Source: CAD feature listing. Evaluate the final solid. Frame: model axes, mm. A direction names the side the tool comes from. Round coordinates to 2 decimals unless told otherwise and drop trailing zeros. Loops run counter-clockwise (first coordinate to the right, second up) from the corner with the lowest first, then second, coordinate; pieces in that order, holes last. Notation, with made-up numbers: M 8,-6.5 L 48,-6.5 A23 cw 48,13.5 Z; hole C -10,62.25 d8. An arc over 180 degrees is marked long. Write each question's results on one line, items separated by ' | '. Start each with the question number.
1. Contact query for flat-ended pins moving along their axis: pin 1 Ø20 at (x, z) = (-3, 4) entering from +Y; pin 2 Ø17.5 at (x, z) = (-15, 15) entering from -Y; pin 3 Ø10 at (y, z) = (-3, 30.5) entering from +X; pin 4 Ø1 at (y, z) = (1, 3.5) entering from -X. Output: stop coordinate, or through.
2. Section A-A on z = 30. Output: boundary loops of the cut face in (x, y).
3. Draft query along Y for faces 5 (the flat face through (0, -9.4, 0)), 6 (the flat face through (-11, 5, 61)), 7 (the cylindrical face through (-1.472, -8.137, 4.674)), 8 (the flat face through (-11, -5, 61)). Return one class per face: released by +Y, released by -Y, zero draft, split by the parting line, or undercut.
4. Section B-B on x = -7. Output: boundary loops of the cut face in (y, z).
5. Set-up query: faces 1 (the flat face through (-2.92, 0.13, 17)), 2 (the flat face through (-8.988, 0.071, 13.305)), 3 (the flat face through (1, 0, 70)), 4 (the cylindrical face through (1.472, 7.763, 4.674)). Return all of +Z, -Z, +X, -X, +Y, -Y with unobstructed straight access to the full face (end or side cutting, diameter ignored); none if empty.
6. Ray query, line 1 (Y direction, x = -5.5, z = 16); line 2 (Y direction, x = -20, z = 50); line 3 (X direction, y = -6.6, z = 30). Return the intervals inside material, ascending.
7. Section C-C on z = 0. Output: boundary loops of the cut face in (x, y), and give its area (3 significant figures).
from build123d import *
from build123d.topology import SkipClean

# Parameters (mm, degrees)
EXTRUDE_1_DEPTH          = 6.8
SKETCH_2_R               = 10
EXTRUDE_1_2_DEPTH        = 14
EXTRUDE_START            = -9
EXTRUDE_2_DEPTH          = 18
CUT_EXTRUDE_1_DEPTH      = 5.1
SKETCH_5_R               = 4.9
EXTRUDE_3_DEPTH          = 15
SKETCH_6_R               = 5.15
CUT_EXTRUDE_5_DEPTH      = 20
CUT_EXTRUDE_8_DEPTH      = 5
CUT_EXTRUDE_8_DEPTH_BACK = 5
CUT_EXTRUDE_8_START      = -9
SKETCH_9_R               = 5.15
CUT_EXTRUDE_9_DEPTH      = 5
SKETCH_11_R              = 0.75
CUT_EXTRUDE_10_DEPTH     = 2
CUT_EXTRUDE_11_DEPTH     = 2
CUT_EXTRUDE_12_DEPTH     = 2
SKETCH_7_W               = 20.220207393
SKETCH_7_H               = 10
CUT_EXTRUDE_14_DEPTH     = 14
CHAMFER_C0_3_SIZE        = 0.3
SKETCH_19_R              = 4.9
EXTRUDE_9_8_2_2_DEPTH    = 2.2
CHAMFER_C0_3_2_SIZE      = 0.3


# Read off the part's stored shape, not the designer's step: the extrude step
with BuildPart() as part:
    # Sketch 1 → Extrude 1 (new, symmetric)
    with BuildSketch(Plane(origin=(0, 0, 0), x_dir=(1, 0, 0), z_dir=(0, 1, 0))):
        Polygon((-5.82435206, 3.882901374), (-27, -27.880570536), (-27, -58.585636208), (0.909866919, -78.68074039), (9.090133081, -67.31925961), (-13, -51.414363792), (-13, -32.119429464), (5.82435206, -3.882901374), align=None)
    extrude(amount=EXTRUDE_1_DEPTH, both=True)

    # Sketch 2 → Extrude 1 2 (add)
    with BuildSketch(Plane(origin=(0, 6.8, 0), x_dir=(1, 0, 0), z_dir=(0, 1, 0))):
        with Locations(Location((0, 0, 0), (0, 0, 270))):
            Circle(SKETCH_2_R)
        with Locations(Location((-20, -30, 0), (0, 0, 270))):
            Circle(SKETCH_2_R)
    extrude(amount=-EXTRUDE_1_2_DEPTH)

    # Extrude 2 outline → Extrude 2 (add)
    with SkipClean():  # the faces are left unmerged after this step: merging them gives an invalid solid
        with BuildSketch(Plane(origin=(0, 0, 0), x_dir=(1, 0, 0), z_dir=(0, 1, 0)).offset(EXTRUDE_START)):
            with BuildLine():
                Line((-14.730348136, -9.47609274), (-21.86300031, -20.175071))
                ThreePointArc((-21.86300031, -20.175071), (-29.570920265, -27.102158513), (-27, -37.141428429))
                Line((-27, -37.141428429), (-27, -58.585636208))
                Line((-27, -58.585636208), (0.909866919, -78.68074039))
                Line((0.909866919, -78.68074039), (9.090133081, -67.31925961))
                Line((9.090133081, -67.31925961), (-13, -51.414363792))
                Line((-13, -51.414363792), (-13, -37.141428429))
                ThreePointArc((-13, -37.141428429), (-10.429079735, -32.897841487), (-10.214296189, -27.940873748))
                Line((-10.214296189, -27.940873748), (-3.081644015, -17.241895487))
                Line((-3.081644015, -17.241895487), (-14.730348136, -9.47609274))
            make_face()
        extrude(amount=EXTRUDE_2_DEPTH)
    add(part.part.scale(1), mode=Mode.REPLACE)  # the faces are merged on a copy

    # Sketch 4 → Cut-Extrude 1 (cut, symmetric)
    with BuildSketch(Plane(origin=(0, 0, 0), x_dir=(1, 0, 0), z_dir=(0, 1, 0))):
        with BuildLine():
            Line((-13, -37.141428429), (-13, -43.141428429))
            Line((-13, -43.141428429), (-27, -43.141428429))
            Line((-27, -43.141428429), (-27, -37.141428429))
            ThreePointArc((-27, -37.141428429), (-29.570920265, -27.102158513), (-21.86300031, -20.175071))
            Line((-21.86300031, -20.175071), (-14.730348136, -9.47609274))
            Line((-14.730348136, -9.47609274), (-3.081644015, -17.241895487))
            Line((-3.081644015, -17.241895487), (-10.214296189, -27.940873748))
            ThreePointArc((-10.214296189, -27.940873748), (-10.429079735, -32.897841487), (-13, -37.141428429))
        make_face()
    extrude(amount=CUT_EXTRUDE_1_DEPTH, both=True, mode=Mode.SUBTRACT)

    # Sketch 5 → Extrude 3 (add)
    with SkipClean():  # the faces are left unmerged after this step: merging them gives an invalid solid
        with BuildSketch(Plane(origin=(0, 9, 0), x_dir=(1, 0, 0), z_dir=(0, 1, 0))):
            with Locations(Location((0, 0, 0), (0, 0, 270))):
                Circle(SKETCH_5_R)
        extrude(amount=-EXTRUDE_3_DEPTH)

    # Sketch 6 → Cut-Extrude 5 (cut)
    with SkipClean():  # the faces are left unmerged after this step: merging them gives an invalid solid
        with BuildSketch(Plane(origin=(0, 9, 0), x_dir=(1, 0, 0), z_dir=(0, 1, 0))):
            with Locations(Location((-20, -30, 0), (0, 0, 270))):
                Circle(SKETCH_6_R)
        extrude(amount=-CUT_EXTRUDE_5_DEPTH, mode=Mode.SUBTRACT)

    # Sketch 8 → Cut-Extrude 8 (cut, two sides: drawn at the far end of the back side and taken through both)
    with SkipClean():  # the faces are left unmerged after this step: merging them gives an invalid solid
        with BuildSketch(Plane(origin=(0, 9, 0), x_dir=(1, 0, 0), z_dir=(0, 1, 0)).offset(CUT_EXTRUDE_8_START - CUT_EXTRUDE_8_DEPTH_BACK)):
            Polygon((3.409392691, -63.229126529), (-4.186568745, -73.779072968), (-26, -58.073402464), (-26, -48.414363792), (-13, -48.414363792), (-13, -51.414363792), align=None)
        extrude(amount=CUT_EXTRUDE_8_DEPTH + CUT_EXTRUDE_8_DEPTH_BACK, mode=Mode.SUBTRACT)

    # Sketch 9 → Cut-Extrude 9 (cut)
    with SkipClean():  # the faces are left unmerged after this step: merging them gives an invalid solid
        with BuildSketch(Plane(origin=(37.908324552, 0, 27.293993678), x_dir=(0.5843047258450756, 0, -0.8115343414514946), z_dir=(0.8115343414514946, 0, 0.5843047258450756))):
            with Locations((-56.320483297, 0)):
                Circle(SKETCH_9_R)
        extrude(amount=-CUT_EXTRUDE_9_DEPTH, mode=Mode.SUBTRACT)

    # Sketch 11 → Cut-Extrude 10 (cut)
    with SkipClean():  # the faces are left unmerged after this step: merging them gives an invalid solid
        with BuildSketch(Plane(origin=(33.850652845, 0, 24.372470048), x_dir=(0.5843047258450756, 0, -0.8115343414514947), z_dir=(0.8115343414514947, 0, 0.5843047258450756))):
            with Locations((-56.320483297, 2.8)):
                Circle(SKETCH_11_R)
            with Locations((-56.320483297, -2.8)):
                Circle(SKETCH_11_R)
        extrude(amount=-CUT_EXTRUDE_10_DEPTH, mode=Mode.SUBTRACT)

    # Sketch 12 → Cut-Extrude 11 (cut)
    with SkipClean():  # the faces are left unmerged after this step: merging them gives an invalid solid
        with BuildSketch(Plane(origin=(0, 9, 0), x_dir=(1, 0, 0), z_dir=(0, 1, 0))):
            Polygon((-14.730348136, -9.47609274), (-3.081644015, -17.241895487), (-8.628645977, -25.56239843), (-20.277350098, -17.796595683), align=None)
        extrude(amount=-CUT_EXTRUDE_11_DEPTH, mode=Mode.SUBTRACT)

    # Sketch 13 → Cut-Extrude 12 (cut)
    with SkipClean():  # the faces are left unmerged after this step: merging them gives an invalid solid
        with BuildSketch(Plane.XZ.offset(9)):
            Polygon((-14.730348136, 9.47609274), (-3.081644015, 17.241895487), (-8.628645977, 25.56239843), (-20.277350098, 17.796595683), align=None)
        extrude(amount=-CUT_EXTRUDE_12_DEPTH, mode=Mode.SUBTRACT)

    # Sketch 7 → Cut-Extrude 14 (cut)
    with BuildSketch(Plane(origin=(-28.818191471, 0, 40.025265932), x_dir=(-0.8115343414514946, 0, -0.5843047258450756), z_dir=(0.5843047258450756, 0, -0.8115343414514946))):
        with Locations((-29.601812998, 0)):
            Rectangle(SKETCH_7_W, SKETCH_7_H)
    extrude(amount=-CUT_EXTRUDE_14_DEPTH, mode=Mode.SUBTRACT)

    # Chamfer C0.3
    chamfer_c0_3_edges = [part.edges().sort_by_distance(p)[0] for p in [
        (0, 9, -4.9),
    ]]
    chamfer(chamfer_c0_3_edges, length=CHAMFER_C0_3_SIZE)

    # Sketch 19 → Extrude 9.8__2.2 (add)
    with BuildSketch(Plane.XZ.offset(7.2)):
        with Locations(Location((0, 0, 0), (0, 0, 90))):
            Circle(SKETCH_19_R)
    extrude(amount=EXTRUDE_9_8_2_2_DEPTH)

    # Chamfer C0.3 2
    chamfer_c0_3_2_edges = [part.edges().sort_by_distance(p)[0] for p in [
        (0, -9.4, -4.9),
    ]]
    chamfer(chamfer_c0_3_2_edges, length=CHAMFER_C0_3_2_SIZE)


solid = part.part
Taken from the geometry:
1) pin 1: y = 9 | pin 2: y = -9 | pin 3: x = -8.9 | pin 4: x = -11.08
2) outline: M -30,-9 L -25.15,-9 L -25.15,-5.1 L -30,-5.1 Z; M -30,5.1 L -25.15,5.1 L -25.15,9 L -30,9 Z; M -14.85,-9 L -10,-9 L -10,-5.1 L -14.85,-5.1 Z; M -14.85,5.1 L -10,5.1 L -10,9 L -14.85,9 Z
3) face 5: released by -Y | face 6: undercut | face 7: zero draft | face 8: undercut
4) outline: M -9,55.73 L -5,55.73 L -5,72.99 L -9,72.99 Z; M -7.2,-7.14 L 6.8,-7.14 L 6.8,14.63 L 7,14.63 L 7,23.12 L 5.1,23.12 L 5.1,14.63 L -5.1,14.63 L -5.1,23.12 L -7,23.12 L -7,14.63 L -6.8,14.63 L -6.8,7.14 L -7.2,7.14 Z; M 5,55.73 L 9,55.73 L 9,72.99 L 5,72.99 Z
5) face 1: +X, +Y, -Y | face 2: -X | face 3: none | face 4: +Y
6) line 1: -7 to -5.1, 5.1 to 7 | line 2: -9 to -5, 5 to 9 | line 3: -30 to -25.15, -14.85 to -10
7) outline: M -10,-7.2 L -4.9,-7.2 L -4.9,-9.1 L -4.6,-9.4 L 4.6,-9.4 L 4.9,-9.1 L 4.9,-7.2 L 10,-7.2 L 10,6.8 L 4.9,6.8 L 4.9,8.7 L 4.6,9 L -4.6,9 L -4.9,8.7 L -4.9,6.8 L -10,6.8 Z | area: 323 mm^2
